The drawing under review shows one solid part. Ordinate dimensions are in mm from its lowest x, y, z. Round coordinates to 2 decimals unless told otherwise and drop trailing zeros. Order: outer loops, then holes, each group sorted by start corner. A loop starts at its lowest first (then second) coordinate and runs counter-clockwise, first axis right, second up.
1) Consider section B-B (y = 36). Give the boundary of the cut face in (x, z), then the cut area to 3 significant figures.
2) To check wall thickness, follow L1, parallel to Y at x = 21.44, z = 0.6; L2, parallel to Y at x = 3, z = 0.4; L3, parallel to Y at x = 15.5, z = 0.25 (1 decimal). State the ranges of each line that lie inside material, in increasing order.
3) Consider section D-D (x = 31.5). Give the boundary of the cut face in (y, z), then the cut area to 3 significant figures.
4) Consider section C-C (z = 0.5). Give the boundary of the cut face in (x, y) (3 decimals), then the cut area to 3 significant figures.
5) Consider section A-A (x = 21.44). Give the boundary of the cut face in (y, z), then the cut area to 3 significant figures.
6) Clearance check with a flat-ended pin moving along its axis: P1, Ø2, axis at x = 3, y = 3, coming from the +Z side. State where the tip first meets the part, or that it passes through.
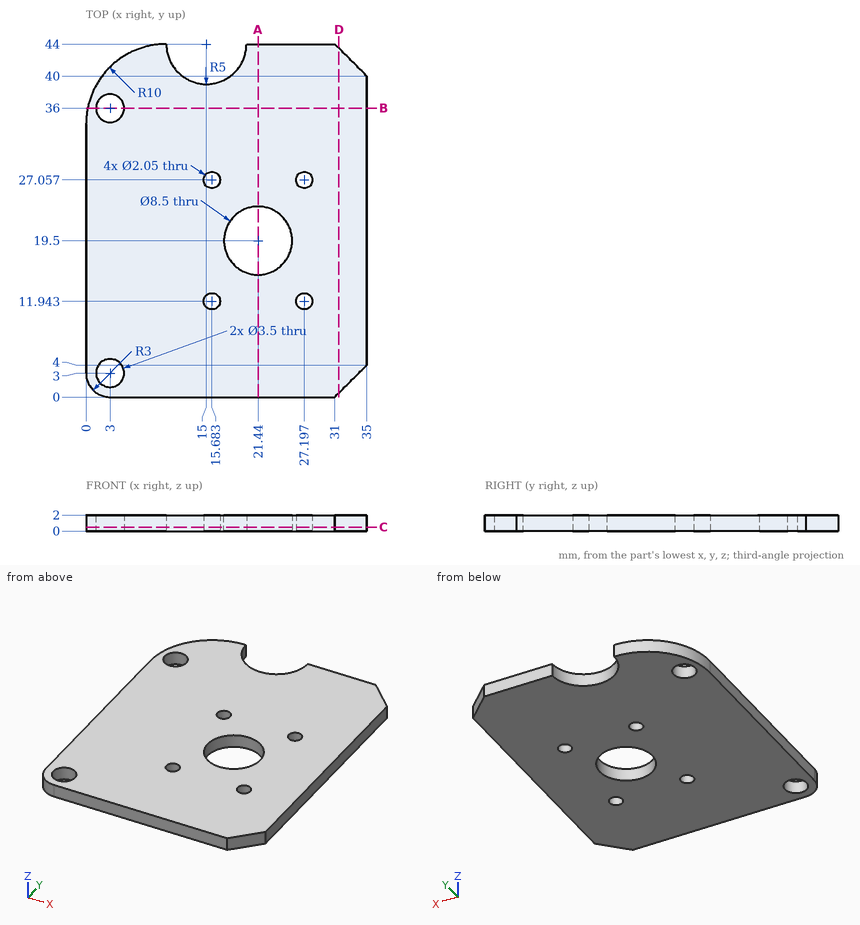
Answer below:
1. outline: (0.2, 0) - (1.25, 0) - (1.25, 2) - (0.2, 2) - close; (4.75, 0) - (35, 0) - (35, 2) - (4.75, 2) - close
1. area: 62.6 mm2
2. L1: y = 0 to 15.25, 23.75 to 44
2. L2: y = 0 to 1.25, 4.75 to 34.25, 37.75 to 41.14
2. L3: y = 0 to 10.9, 13 to 26, 28.1 to 39
3. outline: (0.5, 0) - (43.5, 0) - (43.5, 2) - (0.5, 2) - close
3. area: 86.0 mm2
4. outline: (0, 3) arc R3 ccw to (3, 0) - (31, 0) - (35, 4) - (35, 40) - (31, 44) - (20, 44) arc R5 cw to (10, 44) arc R10 ccw to (0, 34) - close; hole circle Ø3.5 at (3, 3); hole circle Ø3.5 at (3, 36); hole circle Ø2.05 at (15.683, 11.943); hole circle Ø2.05 at (15.683, 27.057); hole circle Ø8.5 at (21.44, 19.5); hole circle Ø2.05 at (27.197, 11.943); hole circle Ø2.05 at (27.197, 27.057)
4. area: 1,370 mm2
5. outline: (0, 0) - (15.25, 0) - (15.25, 2) - (0, 2) - close; (23.75, 0) - (44, 0) - (44, 2) - (23.75, 2) - close
5. area: 71.0 mm2
6. P1: passes through
